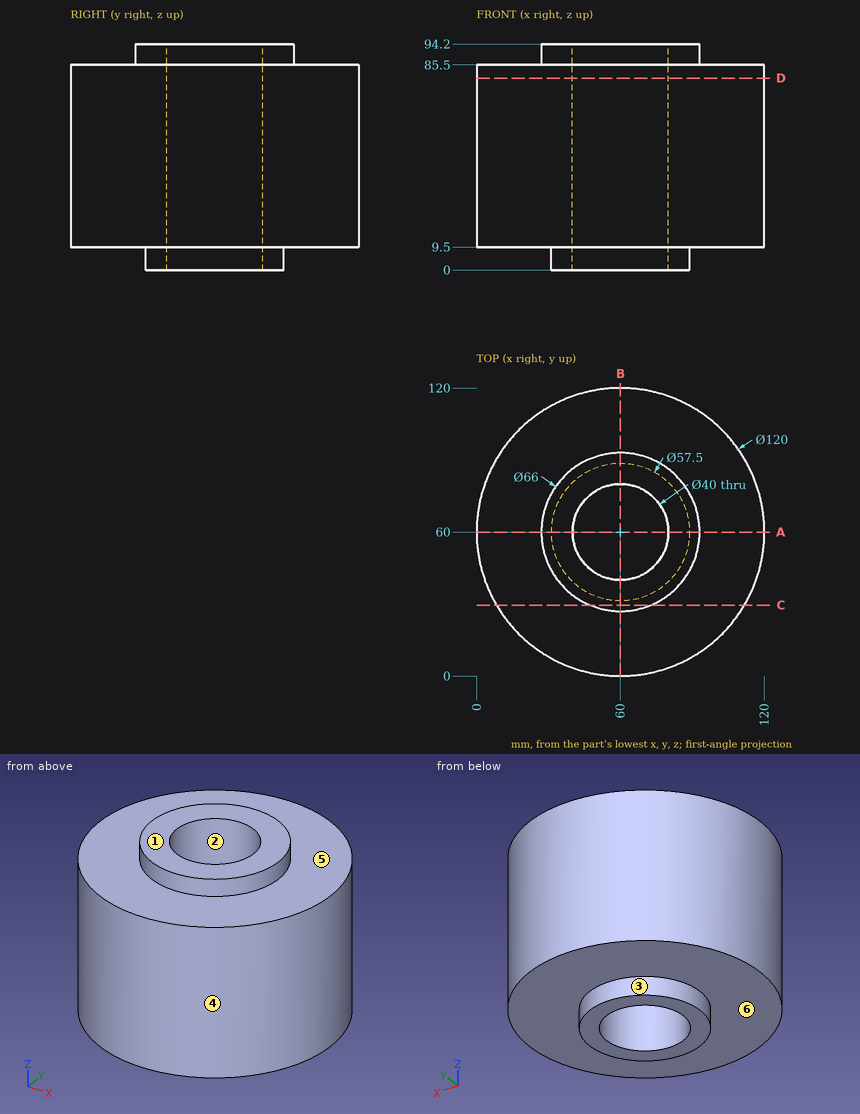
Could you check a few things on this drawing? It's one solid part, dimensions in mm from its lowest x, y, z. A direction names the side the tool comes from. Give positions to 0.01 mm unless a question says otherwise; leave off trailing zeros. Write each loop counter-clockwise with the first axis right and the second up, starting at its lowest first coordinate (ties: lowest second). Pieces come first, ordered by that corner, then holes. Notation, with made-up numbers: (76.25, -19.5) -> (105.25, -19.5) arc R31 ccw to (105.25, 8.5) -> close; hole circle Ø4 at (28.25, 0). An arc over 180 degrees is marked (long way). Write item = value, one per line.
(1) Suppose I cut it at C-C on y = 29.5. Write out the boundary of the cut face in (x, z).
Worked out:
outline = (8.33, 9.5) -> (111.67, 9.5) -> (111.67, 85.5) -> (72.6, 85.5) -> (72.6, 94.2) -> (47.4, 94.2) -> (47.4, 85.5) -> (8.33, 85.5) -> close
(2) I'm going to push flat-ended pins straight in: P1, Ø1.5, axis at y = 15, z = 22.5, coming from the +X side; P2, Ø12, axis at y = 94, z = 61, coming from the +X side; P3, Ø3, axis at x = 28.5, y = 98, coming from the +Z side. Where does each tip first touch, or does it pass through?
Worked out:
P1 = 100.52
P2 = 113.07
P3 = 85.5
(3) For the marked faces 4, 5 and 6, which set-ups out of +Z, -Z, +X, -X, +Y, -Y let a thin tool reach every point of the face, with its end or its side?
Worked out:
face_4 = +Z, -Z
face_5 = +Z
face_6 = -Z
(4) Suppose I cut it at A-A on y = 60. Write out the boundary of the cut face in (x, z), then the cut area to 3 significant figures.
Worked out:
outline = (0, 9.5) -> (31.25, 9.5) -> (31.25, 0) -> (40, 0) -> (40, 94.2) -> (27, 94.2) -> (27, 85.5) -> (0, 85.5) -> close; (80, 0) -> (88.75, 0) -> (88.75, 9.5) -> (120, 9.5) -> (120, 85.5) -> (93, 85.5) -> (93, 94.2) -> (80, 94.2) -> close
area = 6,470 mm^2
(5) Thinking about a two-plate mould opening in X: for the marked faces 1, 2 and 3, which applies, released by +X, released by -X, zero draft, split by the parting line, or undercut?
Worked out:
face_1 = zero draft
face_2 = undercut
face_3 = split by the parting line
(6) Suppose I cut it at D-D on z = 80. Write out the boundary of the cut face in (x, y).
Worked out:
outline = circle Ø120 at (60, 60); hole circle Ø40 at (60, 60)
(7) I need wall thicknesses on probe 1 along X at (y, z) = (59.5, 70); probe 2 along Y at (x, z) = (60, 42.5); probe 3 along Z at (x, y) = (25, 103). Which ranges of each line are inside material? Lowest first, please. Write a range as from..to.
Worked out:
probe_1 = 0..40.01, 79.99..120
probe_2 = 0..40, 80..120
probe_3 = 9.5..85.5
